CAD build for the part. Positions are in the model's coordinates, mm. Face numbers are marked on the shaded views. A direction names the side the tool comes from. Coordinates: 2 decimals unless noted, no trailing zeros. Order: outer loops, then holes, each group sorted by start corner. A loop starts at its lowest first (then second) coordinate and runs counter-clockwise, first axis right, second up. Notation, with made-up numbers: (-1.5, -27) - (20.5, -27) arc R26 ccw to (20.5, 7) - close; hole circle Ø10 at (22, -18.5). An arc over 180 degrees is marked (long way). Return JSON: item names as keys, results as strings.
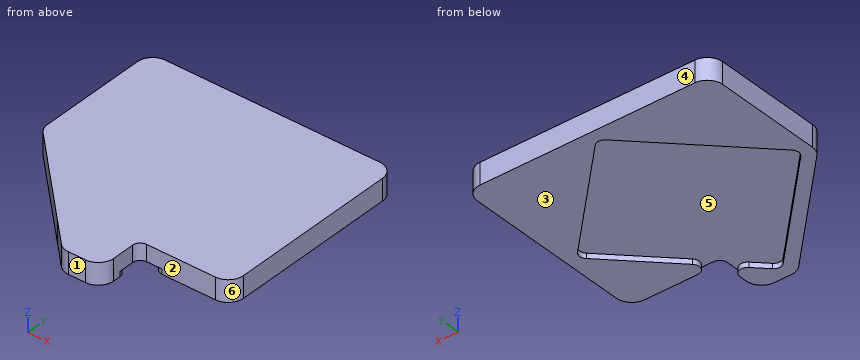
from build123d import *

# Parameters (mm, degrees)
F1_DEPTH = 1.4
F2_START = 0.33
F2_DEPTH = 1.07
F3_R     = 1
F4_F1_R  = 0.5
F4_F2_R  = 0.5


# Not quite as in the source:
# - two fillets or chamfers of one size are made in one step
# - a feature names something its author has since deleted; it is built from what else it names


with BuildPart() as f1:
    # F0 (on Top) → F1 (new body)
    with BuildSketch(Plane.XY):
        Polygon((5.6168799675, 1.8509632612), (7.4634256667, 0), (10, 0), (10, 2.6923049909), (7.9488945061, 0.6460947242), (0.6037752352, 8.0087860049), (7.9664665159, 15.3539052758), (15.3115857869, 7.9912139951), (10.3084311196, 3), (16, 3), (16, 16), (0, 16), (0, 7.4812807055), (2.1561987725, 5.3199235762), align=None)
    extrude(amount=F1_DEPTH)

    # F0 (on Top) → F2 (join)
    with BuildSketch(Plane.XY.offset(F2_START)):
        Polygon((7.9488945061, 0.6460947242), (10, 2.6923049909), (10, 3), (10.3084311196, 3), (15.3115857869, 7.9912139951), (7.9664665159, 15.3539052758), (0.6037752352, 8.0087860049), align=None)
    extrude(amount=F2_DEPTH)

    # F3
    f3_edges = [f1.edges().sort_by_distance(p)[0] for p in [
        (16, 16, 0.7),
        (0, 16, 0.7),
        (10, 0, 0.7),
        (16, 3, 0.7),
        (0, 7.481281, 0.7),
        (7.463426, 0, 0.7),
    ]]
    fillet(f3_edges, radius=F3_R)

    # F4: fillet of radius 0.5 on 7 edges, made by hand

    # F4_f1
    f4_f1_edges = [f1.edges().sort_by_distance(p)[0] for p in [
        (10.3084311196, 3, 0.165),
        (10, 2.6923049909, 0.165),
    ]]
    fillet(f4_f1_edges, radius=F4_F1_R)

    # F4_f2
    f4_f2_edges = [f1.edges().sort_by_distance(p)[0] for p in [
        (7.9664665159, 15.3539052758, 0.165),
        (0.6037752352, 8.0087860049, 0.165),
        (7.9488945061, 0.6460947242, 0.165),
        (15.3115857869, 7.9912139951, 0.165),
        (10, 3, 0.865),
    ]]
    fillet(f4_f2_edges, radius=F4_F2_R)


solid = f1.part
Item 1: Band-saw the part on C-C, the plane x = 12.25. List the corners of the cut face in (y, z), then the cut area to 3 significant figures.
Findings below:
{"outline": "(3, 0) - (4.94, 0) - (4.94, 0.33) - (11.06, 0.33) - (11.06, 0) - (16, 0) - (16, 1.4) - (3, 1.4) - close", "area": "16.2 mm²"}
Item 2: Band-saw the part on A-A, the plane z = 0.8. List the corners of the cut face in (x, y), then the cut area to 3 significant figures.
Findings below:
{"outline": "(0, 7.89) arc R1 ccw to (0.29, 7.19) - (7.17, 0.29) arc R1 ccw to (7.88, 0) - (9, 0) arc R1 ccw to (10, 1) - (10, 2.5) arc R0.5 cw to (10.5, 3) - (15, 3) arc R1 ccw to (16, 4) - (16, 15) arc R1 ccw to (15, 16) - (1, 16) arc R1 ccw to (0, 15) - close", "area": "209 mm²"}
Item 3: Which spindle directions (+Z, -Z, +X, -X, +Y, -Y) get a long thin tool onto all of the face, cutting with end or side? Do the marked faces 1 and 2. Say none if no direction does.
Findings below:
{"face 1": "+Z, -Z, +X, -X, -Y", "face 2": "+Z, -Z, +X, -Y"}
Item 4: Mould opens along Y. For the marked faces 3, 4, 5 and 6 say: released by +Y, released by -Y, zero draft, split by the parting line, or undercut.
Findings below:
{"face 3": "zero draft", "face 4": "released by +Y", "face 5": "undercut", "face 6": "released by -Y"}
Item 5: Wall check: L1, parallel to Y at x = 11.5, z = 1.05; L2, parallel to Z at x = 8, y = 6.75; L3, parallel to Y at x = 2.5, z = 0.25. Give the ranges that are in metal, low to high. Write a range as [from, to].
Findings below:
{"L1": "y = [3, 16]", "L2": "z = [0.33, 1.4]", "L3": "y = [4.98, 6.11], [9.9, 16]"}
Item 6: Band-saw the part on B-B, the plane y = 10.25. List the corners of the cut face in (x, z), then the cut area to 3 significant figures.
Findings below:
{"outline": "(0, 0) - (2.85, 0) - (2.85, 0.33) - (13.06, 0.33) - (13.06, 0) - (16, 0) - (16, 1.4) - (0, 1.4) - close", "area": "19.0 mm²"}
